Geometry check sheet. Reference: the model listing, model coordinates, mm. Face numbers are marked on the shaded views. A direction names the side the tool comes from. Coordinates: 2 decimals unless noted, no trailing zeros. Loops run counter-clockwise (first coordinate to the right, second up) from the corner with the lowest first, then second, coordinate; pieces in that order, holes last.
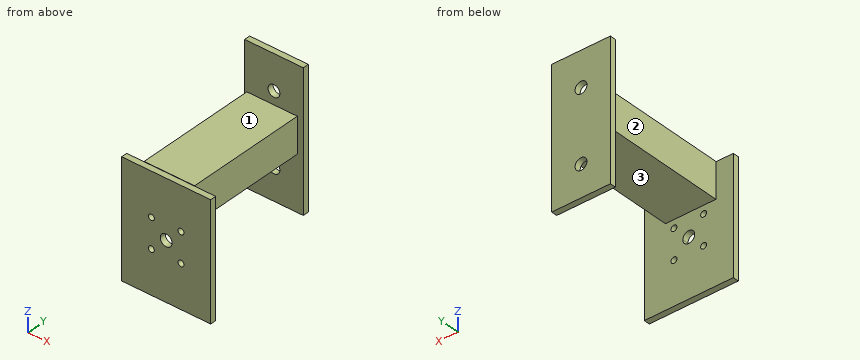
from build123d import *

# Parameters (mm, degrees)
SKETCH_1_R      = 1
EXTRUDE_1_DEPTH = 2
SKETCH_2_W      = 17.022580328
SKETCH_2_H      = 11.892604249
EXTRUDE_2_DEPTH = 43
EXTRUDE_START   = -2
SKETCH_3_W      = 19.786200008
SKETCH_3_H      = 46.373293121
SKETCH_3_R      = 2
EXTRUDE_3_DEPTH = 2


with BuildPart() as part:
    # Sketch 1 → Extrude 1 (new body)
    # profile 1 of 2: a face of its own
    with BuildSketch(Plane(origin=(0, 0, 0), x_dir=(1, 0, 0), z_dir=(0, 1, 0))):
        with BuildLine():
            ThreePointArc((7.25, 19.5), (9.25, 21.5), (11.25, 19.5))
            Line((11.25, 19.5), (24.25, 19.5))
            Line((24.25, 19.5), (24.25, 39))
            Line((24.25, 39), (0, 39))
            Line((0, 39), (-5.75, 39))
            Line((-5.75, 39), (-5.75, 19.5))
            Line((-5.75, 19.5), (7.25, 19.5))
        make_face()
        with Locations(Location((4.25, 24.5, 0), (0, 0, 270))):
            Circle(SKETCH_1_R, mode=Mode.SUBTRACT)
        with Locations(Location((14.25, 24.5, 0), (0, 0, 270))):
            Circle(SKETCH_1_R, mode=Mode.SUBTRACT)
    # profile 2 of 2: a face of its own
    with BuildSketch(Plane(origin=(0, 0, 0), x_dir=(1, 0, 0), z_dir=(0, 1, 0))):
        with BuildLine():
            Line((24.25, 19.5), (11.25, 19.5))
            ThreePointArc((11.25, 19.5), (10.664213562, 18.085786438), (9.25, 17.5))
            ThreePointArc((9.25, 17.5), (7.835786438, 18.085786438), (7.25, 19.5))
            Line((7.25, 19.5), (-5.75, 19.5))
            Line((-5.75, 19.5), (-5.75, 0))
            Line((-5.75, 0), (0, 0))
            Line((0, 0), (24.25, 0))
            Line((24.25, 0), (24.25, 19.5))
        make_face()
        with Locations(Location((4.25, 14.5, 0), (0, 0, 270))):
            Circle(SKETCH_1_R, mode=Mode.SUBTRACT)
        with BuildLine():
            ThreePointArc((15.25, 14.5), (14.25, 13.5), (13.25, 14.5))
            ThreePointArc((13.25, 14.5), (14.25, 15.5), (15.25, 14.5))
        make_face(mode=Mode.SUBTRACT)
    extrude(amount=EXTRUDE_1_DEPTH)

    # Sketch 2 → Extrude 2 (add)
    with BuildSketch(Plane(origin=(0, 2, 0), x_dir=(1, 0, 0), z_dir=(0, 1, 0))):
        with Locations((8.624620537, 5.830652978)):
            Rectangle(SKETCH_2_W, SKETCH_2_H)
    extrude(amount=EXTRUDE_2_DEPTH)

    # Sketch 3 → Extrude 3 (add)
    with BuildSketch(Plane(origin=(0, 45, 0), x_dir=(1, 0, 0), z_dir=(0, 1, 0)).offset(EXTRUDE_START)):
        with Locations((9.25, 6.951413881)):
            Rectangle(SKETCH_3_W, SKETCH_3_H)
        with Locations(Location((9.25, -4.5, 0), (0, 0, 270))):
            Circle(SKETCH_3_R, mode=Mode.SUBTRACT)
        with Locations(Location((9.25, 19.5, 0), (0, 0, 270))):
            Circle(SKETCH_3_R, mode=Mode.SUBTRACT)
    extrude(amount=EXTRUDE_3_DEPTH)


solid = part.part
(1) Sectioned sample at C-C on z = -8. Record the cut outline in (x, y).
Findings:
outline: (-5.75, 0) - (24.25, 0) - (24.25, 2) - (17.14, 2) - (17.14, 43) - (19.14, 43) - (19.14, 45) - (-0.64, 45) - (-0.64, 43) - (0.11, 43) - (0.11, 2) - (-5.75, 2) - close
(2) Gauge pin test, flat ends, axial feed: pin 1 Ø9.5 at (y, z) = (22, -8.5) entering from +X; pin 2 Ø5 at (x, y) = (5, 18.5) entering from -Z; pin 3 Ø1.6 at (y, z) = (43.5, -7.5) entering from -X. Record the tip position at first contact, or that the pin passes through.
Findings:
pin 1: stops at x = 17.14
pin 2: stops at z = -11.78
pin 3: stops at x = -0.64
(3) Sectioned sample at A-A on z = -14.5. Record the cut outline in (x, y).
Findings:
outline: (-5.75, 0) - (3.25, 0) - (3.25, 2) - (-5.75, 2) - close; (-0.64, 43) - (19.14, 43) - (19.14, 45) - (-0.64, 45) - close; (5.25, 0) - (13.25, 0) - (13.25, 2) - (5.25, 2) - close; (15.25, 0) - (24.25, 0) - (24.25, 2) - (15.25, 2) - close
(4) Sectioned sample at D-D on y = 40.5. Record the cut outline in (x, z).
Findings:
outline: (0.11, -11.78) - (17.14, -11.78) - (17.14, 0.12) - (0.11, 0.12) - close
(5) Scan lines: L1, parallel to Y at x = 2.5, z = -20; L2, parallel to X at y = 44.05, z = -19.5; L3, parallel to Z at x = 13.5, y = 22.5. Record each from-to range of solid material in increasing order.
Findings:
L1: y = 0 to 2, 43 to 45
L2: x = -0.64 to 7.25, 11.25 to 19.14
L3: z = -11.78 to 0.12
(6) Sectioned sample at B-B on x = 14.25. Record the cut outline in (y, z).
Findings:
outline: (0, -39) - (2, -39) - (2, -25.5) - (0, -25.5) - close; (0, -23.5) - (2, -23.5) - (2, -15.5) - (0, -15.5) - close; (0, -13.5) - (2, -13.5) - (2, -11.78) - (43, -11.78) - (43, -30.14) - (45, -30.14) - (45, 16.24) - (43, 16.24) - (43, 0.12) - (2, 0.12) - (2, 0) - (0, 0) - close
(7) Access from +Z, -Z, +X, -X, +Y, -Y to the whole of each face (thin tool, end or side, straight path). Record for the marked faces 1, 2 and 3.
Findings:
face 1: +Z, +X, -X, -Y
face 2: +Z, -Z, -X
face 3: -Z, +X, -X
